```python
from build123d import *

# Parameters (mm, degrees)
F1_DEPTH  = 34
F2_W      = 9
F2_H      = 9
F3_DEPTH  = 5
F4_R      = 3.5
F5_DEPTH  = 6
F6_W      = 5
F6_H      = 9.5
F7_DEPTH  = 4
F8_W      = 20.85
F8_H      = 14
F9_DEPTH  = 34.001
F10_W     = 5
F10_H     = 14
F11_DEPTH = 6
F12_W     = 5
F12_H     = 14
F13_DEPTH = 6
F15_DEPTH = 3.5


with BuildPart() as f1:
    # F0 (on Front) → F1 (new body)
    with BuildSketch(Plane.XZ):
        Polygon((0.85, 13), (-25, 13), (-25, -13), (25, -13), (25, 3), (20, 3), (20, -1), (0.85, -1), align=None)
    extrude(amount=F1_DEPTH)

    # F2 (on face) → F3 (cut, through all)
    with BuildSketch(Plane.YZ.offset(25)):
        with Locations((-16.5, -1.5)):
            Rectangle(F2_W, F2_H)
    extrude(amount=-F3_DEPTH, mode=Mode.SUBTRACT)

    # F4 (on face) → F5 (cut)
    with BuildSketch(Plane(origin=(-25, 0, 0), x_dir=(0, -1, 0), z_dir=(-1, 0, 0))):
        with Locations((17, -5)):
            Circle(F4_R)
    extrude(amount=-F5_DEPTH, mode=Mode.SUBTRACT)

    # F6 (on face) → F7 (join, through all)
    with BuildSketch(Plane.XY.offset(-1)):
        with Locations((17.5, -29.25)):
            Rectangle(F6_W, F6_H)
        with Locations((17.5, -4.75)):
            Rectangle(F6_W, F6_H)
    extrude(amount=F7_DEPTH)

    # F8 (on face) → F9 (cut, through all)
    with BuildSketch(Plane.XZ.offset(34)):
        with Locations((-9.575, 6)):
            Rectangle(F8_W, F8_H)
    extrude(amount=-F9_DEPTH, mode=Mode.SUBTRACT)

    # F10 (on face) → F11 (join)
    with BuildSketch(Plane.XZ.offset(34)):
        with Locations((-17.5, 6)):
            Rectangle(F10_W, F10_H)
    extrude(amount=-F11_DEPTH)

    # F12 (on face) → F13 (join)
    with BuildSketch(Plane(origin=(0, 0, 0), x_dir=(-1, 0, 0), z_dir=(0, 1, 0))):
        with Locations((17.5, 6)):
            Rectangle(F12_W, F12_H)
    extrude(amount=-F13_DEPTH)

    # F14 (on face) → F15 (join)
    with BuildSketch(Plane.XY.offset(-1)):
        Polygon((-3, 0), (-15, 0), (-15, -6), (-20, -6), (-20, -28), (-15, -28), (-15, -34), (-3, -34), align=None)
    extrude(amount=F15_DEPTH)


solid = f1.part
```
Work out the finished part from the listing and answer in its coordinate system (mm). A direction names the side the tool comes from. Round coordinates to 2 decimals unless told otherwise and drop trailing zeros. Write each loop counter-clockwise with the first axis right and the second up, starting at its lowest first coordinate (ties: lowest second). Pieces come first, ordered by that corner, then holes. Notation, with made-up numbers: (42.25, 78) - (66.25, 78) arc R12 cw to (66.25, 85) - close; hole circle Ø6 at (30, 39.5). An arc over 180 degrees is marked (long way). Return JSON: item names as keys, results as strings. Group by question number.
Q1. For faces 1 (the flat face through (20, -17, -3)), 2 (the flat face through (-19, -17, -5)), 3 (the flat face through (20, -27, 3)), 4 (the flat face through (-3, -17, 1)), 5 (the flat face through (17, -9.5, 1)), determine the directions among +Z, -Z, +X, -X, +Y, -Y from which every point of the face is accessible in a straight line to the end or side of a thin tool.
Q2. The mould has two halves that part along Y. Classify faces 6 (the flat face through (-25, -17, 0)), 7 (the flat face through (0, 0, -3)), 8 (the flat face through (0, -34, -3)), 9 (the flat face through (17, -24.5, 1)): released by +Y, released by -Y, zero draft, split by the parting line, or undercut.
Q3. The part is cut by section B-B on x = 18. Write down the section's boundary in (y, z), then the cut area to 3 significant figures.
Q4. Each of these flat-tipped pins is pushed along its axis until it touches: pin 1 Ø5 at (x, y) = (-7.5, -24) entering from +Z; pin 2 Ø1 at (y, z) = (-13.5, 0.5) entering from +X; pin 3 Ø6.5 at (y, z) = (-2, 9) entering from +X. Where does it stop, or does it pass through?
Q5. The part is cut by section A-A on z = -5. Write down the section's boundary in (x, y), then the cut area to 3 significant figures.
Q6. The part is cut by section D-D on y = -23. Write down the section's boundary in (x, z), then the cut area to 4 significant figures.
Q7. Find the intervals of material crossed by L1, parallel to Z at x = -22.15, y = -17; L2, parallel to Z at x = 11, y = -28.5; L3, parallel to X at y = -20, z = -3, in increasing order.
Q8. The part is cut by section C-C on y = -17. Write down the section's boundary in (x, z), then the cut area to 4 significant figures.
Solved:
{
 "1": {"face 1": "+Z, +X", "face 2": "-X", "face 3": "+Z, +X, +Y, -Y", "face 4": "+Z, +Y, -Y", "face 5": "+Z"},
 "2": {"face 6": "zero draft", "face 7": "released by +Y", "face 8": "released by -Y", "face 9": "undercut"},
 "3": {"outline": "(-34, -13) - (0, -13) - (0, 3) - (-9.5, 3) - (-9.5, -1) - (-24.5, -1) - (-24.5, 3) - (-34, 3) - close", "area": "484 mm²"},
 "4": {"pin 1": "z = 2.5", "pin 2": "x = -3", "pin 3": "x = -15"},
 "5": {"outline": "(-25, -34) - (25, -34) - (25, -21) - (20, -21) - (20, -12) - (25, -12) - (25, 0) - (-25, 0) - (-25, -13.5) - (-19, -13.5) - (-19, -20.5) - (-25, -20.5) - close", "area": "1,610 mm²"},
 "6": {"outline": "(-25, -13) - (25, -13) - (25, 3) - (20, 3) - (20, -1) - (-3, -1) - (-3, 2.5) - (-20, 2.5) - (-20, 13) - (-25, 13) - close", "area": "749.5 mm²"},
 "7": {"L1": "-13 to -8.5, -1.5 to 13", "L2": "-13 to -1", "L3": "-25 to 20"},
 "8": {"outline": "(-25, -13) - (25, -13) - (25, -6) - (20, -6) - (20, -1) - (-3, -1) - (-3, 2.5) - (-20, 2.5) - (-20, 13) - (-25, 13) - (-25, -1.5) - (-19, -1.5) - (-19, -8.5) - (-25, -8.5) - close", "area": "662.5 mm²"}
}
